from build123d import *

# Parameters (mm, degrees)
F0_W     = 38.1
F0_H     = 38.1
F6_DEPTH = 19.05
F1_R     = 4.35991
F7_DEPTH = 19.05
F2_W     = 6.35
F2_H     = 3.175
F3_W     = 6.35
F3_H     = 3.175
F8_DEPTH = 19.05
F4_R     = 1.5875
F5_R     = 1.5875
F9_DEPTH = 19.05


with BuildPart() as f6:
    # F0 (on Front) → F6 (new body, symmetric)
    with BuildSketch(Plane.XZ):
        Rectangle(F0_W, F0_H)
    extrude(amount=F6_DEPTH, both=True)

    # F1 (on Front) → F7 (cut, symmetric)
    with BuildSketch(Plane.XZ):
        Circle(F1_R)
    extrude(amount=F7_DEPTH, both=True, mode=Mode.SUBTRACT)

    # F2 (on Front) + F3 (on Front) → F8 (cut, through all)
    with BuildSketch(Plane.XZ):
        with Locations((-15.875, -1.5875)):
            Rectangle(F2_W, F2_H)
    with BuildSketch(Plane.XZ):
        with Locations((15.875, -1.5875)):
            Rectangle(F3_W, F3_H)
    extrude(amount=-F8_DEPTH, mode=Mode.SUBTRACT)

    # F4 (on Right) + F5 (on Right) → F9 (cut, symmetric)
    with BuildSketch(Plane.YZ):
        with Locations((0, 12.7)):
            Circle(F4_R)
    with BuildSketch(Plane.YZ):
        with Locations((0, -12.7)):
            Circle(F5_R)
    extrude(amount=F9_DEPTH, both=True, mode=Mode.SUBTRACT)


solid = f6.part
The model under review builds one solid part; all positions refer to its coordinate system, in mm. A direction names the side the tool comes from. Give positions to 0.01 mm unless a question says otherwise; leave off trailing zeros. Write each loop counter-clockwise with the first axis right and the second up, starting at its lowest first coordinate (ties: lowest second). Pieces come first, ordered by that corner, then holes.
1. Tool access review of faces 4 (the flat face through (-16, 9, 0)), 5 (the flat face through (16, 0, -2)), 6 (the cylindrical face through (2.34, -0.27, 3.68)): name each direction out of +Z, -Z, +X, -X, +Y, -Y from which nothing blocks a thin tool from reaching the whole face with its end or side.
2. For P1, Ø1, axis at x = -16, z = -2, coming from the +Y side; P2, Ø1.6, axis at y = 12.5, z = -1.5, coming from the +X side, all flat-tipped, find the tip position at first contact; note any pin that passes through.
3. Add section C-C, the plane x = 16.5. Count the separate pieces of the cut face and the enclosed holes in it, plus the area to 3 significant figures.
4. Add section A-A, the plane y = -1. Write out the cut boundary in (x, z).
5. Add section B-B, the plane z = -12.7. Write out the cut boundary in (x, y), plus the area to 3 significant figures.
6. Wall thickness on L1, parallel to Z at x = -7, y = 0; L2, parallel to Z at x = 15.5, y = 4.5 (3 decimals); L3, parallel to Z at x = 0, y = -14: over which ranges is each line inside the solid? List them lowest first.
7. Draft analysis for pull direction Z (two halves, no side actions). For faces 1 (the flat face through (0, 0, -19.05)), 2 (the flat face through (-16, 0, -2)), 3 (the flat face through (0, 19.05, 5)), state which applies: +Z half, -Z half, draft (parallel to the pull), parting line (faces both ways), or undercut.
8. Add section D-D, the plane y = 7.5. Write out the cut boundary in (x, z) (3 decimals).
Worked answers:
1. face 4: -X, +Y
1. face 5: +X, +Y
1. face 6: +Y, -Y
2. P1: stops at y = 0
2. P2: stops at x = 12.7
3. separate pieces: 1
3. enclosed holes: 2
3. area: 1,380 mm2
4. outline: (-19.05, -19.05) - (19.05, -19.05) - (19.05, -13.93) - (-19.05, -13.93) - close; (-19.05, -11.47) - (19.05, -11.47) - (19.05, 11.47) - (-19.05, 11.47) - close; (-19.05, 13.93) - (19.05, 13.93) - (19.05, 19.05) - (-19.05, 19.05) - close; hole circle Ø8.72 at (0, 0)
5. outline: (-19.05, -19.05) - (19.05, -19.05) - (19.05, -1.59) - (-19.05, -1.59) - close; (-19.05, 1.59) - (19.05, 1.59) - (19.05, 19.05) - (-19.05, 19.05) - close
5. area: 1,330 mm2
6. L1: z = -19.05 to -14.29, -11.11 to 11.11, 14.29 to 19.05
6. L2: z = -19.05 to -3.175, 0 to 19.05
6. L3: z = -19.05 to -4.36, 4.36 to 19.05
7. face 1: -Z half
7. face 2: undercut
7. face 3: draft
8. outline: (-19.05, -19.05) - (19.05, -19.05) - (19.05, -3.175) - (12.7, -3.175) - (12.7, 0) - (19.05, 0) - (19.05, 19.05) - (-19.05, 19.05) - (-19.05, 0) - (-12.7, 0) - (-12.7, -3.175) - (-19.05, -3.175) - close; hole circle Ø8.72 at (0, 0)
